```python
from build123d import *

# Parameters (mm, degrees)
SKETCH1_W           = 75
SKETCH1_H           = 30
BOSS_EXTRUDE1_DEPTH = 8
SKETCH2_R           = 2.5
CUT_EXTRUDE1_DEPTH  = 9
CUT_EXTRUDE2_DEPTH  = 2
FILLET1_R           = 8
SKETCH3_R           = 1.75
CUT_EXTRUDE3_DEPTH  = 25


with BuildPart() as part:
    # Sketch1 → Boss-Extrude1 (new body)
    with BuildSketch(Plane(origin=(0, 0, 0), x_dir=(1, 0, 0), z_dir=(0, 1, 0))):
        with Locations((37.5, 15)):
            Rectangle(SKETCH1_W, SKETCH1_H)
    extrude(amount=BOSS_EXTRUDE1_DEPTH)

    # Sketch2 → Cut-Extrude1 (cut, through all)
    with BuildSketch(Plane(origin=(0, 8, 0), x_dir=(1, 0, 0), z_dir=(0, 1, 0))):
        with Locations((10, 23)):
            Circle(SKETCH2_R)
        with Locations((10, 9)):
            Circle(SKETCH2_R)
        with Locations((65, 23)):
            Circle(SKETCH2_R)
        with Locations((65, 9)):
            Circle(SKETCH2_R)
        with BuildLine():
            Line((15, 28), (60, 28))
            add(Edge.make_bspline(
                [(60, 28), (59.263620849, -4.332136717), (15.33607355, -7.019589548), (15, 28)],
                knots=[0, 0, 0, 0, 1, 1, 1, 1], degree=3))
        make_face()
    extrude(amount=-CUT_EXTRUDE1_DEPTH, mode=Mode.SUBTRACT)

    # Sketch2<3> → Cut-Extrude2 (cut)
    with BuildSketch(Plane(origin=(0, 8, 0), x_dir=(1, 0, 0), z_dir=(0, 1, 0))):
        with BuildLine():
            Line((12.5, 6.5), (12.5, 9))
            ThreePointArc((12.5, 9), (11.767766965, 7.232233059), (10.000000035, 6.5))
            Line((10.000000035, 6.5), (12.5, 6.5))
        make_face()
        with BuildLine():
            Line((12.5, 9), (12.5, 11.5))
            Line((12.5, 11.5), (10, 11.5))
            ThreePointArc((10, 11.5), (11.767766953, 10.767766953), (12.5, 9))
        make_face()
        with BuildLine():
            ThreePointArc((7.5, 9), (8.232233047, 10.767766953), (10, 11.5))
            Line((10, 11.5), (7.5, 11.5))
            Line((7.5, 11.5), (7.5, 9))
        make_face()
        with BuildLine():
            ThreePointArc((10.000000035, 6.5), (8.232233059, 7.232233035), (7.5, 9))
            Line((7.5, 9), (7.5, 6.5))
            Line((7.5, 6.5), (10.000000035, 6.5))
        make_face()
        with BuildLine():
            ThreePointArc((7.5, 23), (8.232233047, 24.767766953), (10, 25.5))
            Line((10, 25.5), (7.5, 25.5))
            Line((7.5, 25.5), (7.5, 23))
        make_face()
        with BuildLine():
            Line((12.5, 23), (12.5, 25.5))
            Line((12.5, 25.5), (10, 25.5))
            ThreePointArc((10, 25.5), (11.767766953, 24.767766953), (12.5, 23))
        make_face()
        with BuildLine():
            Line((12.5, 20.5), (12.5, 23))
            ThreePointArc((12.5, 23), (11.767766953, 21.232233047), (10, 20.5))
            Line((10, 20.5), (12.5, 20.5))
        make_face()
        with BuildLine():
            ThreePointArc((10, 20.5), (8.232233047, 21.232233047), (7.5, 23))
            Line((7.5, 23), (7.5, 20.5))
            Line((7.5, 20.5), (10, 20.5))
        make_face()
        with BuildLine():
            Line((65, 25.5), (62.5, 25.5))
            Line((62.5, 25.5), (62.5, 23))
            ThreePointArc((62.5, 23), (63.232233047, 24.767766953), (65, 25.5))
        make_face()
        with BuildLine():
            Line((67.5, 25.5), (65, 25.5))
            ThreePointArc((65, 25.5), (66.767766953, 24.767766953), (67.5, 23))
            Line((67.5, 23), (67.5, 25.5))
        make_face()
        with BuildLine():
            Line((67.5, 20.5), (67.5, 23))
            ThreePointArc((67.5, 23), (66.767766953, 21.232233047), (65, 20.5))
            Line((65, 20.5), (67.5, 20.5))
        make_face()
        with BuildLine():
            ThreePointArc((65, 20.5), (63.232233047, 21.232233047), (62.5, 23))
            Line((62.5, 23), (62.5, 20.5))
            Line((62.5, 20.5), (65, 20.5))
        make_face()
        with BuildLine():
            Line((67.5, 6.5), (67.5, 9))
            ThreePointArc((67.5, 9), (66.767766953, 7.232233047), (65, 6.5))
            Line((65, 6.5), (67.5, 6.5))
        make_face()
        with BuildLine():
            ThreePointArc((65, 6.5), (63.232233047, 7.232233047), (62.5, 9))
            Line((62.5, 9), (62.5, 6.5))
            Line((62.5, 6.5), (65, 6.5))
        make_face()
        with BuildLine():
            Line((65, 11.5), (62.5, 11.5))
            Line((62.5, 11.5), (62.5, 9))
            ThreePointArc((62.5, 9), (63.232233047, 10.767766953), (65, 11.5))
        make_face()
        with BuildLine():
            Line((67.5, 11.5), (65, 11.5))
            ThreePointArc((65, 11.5), (66.767766953, 10.767766953), (67.5, 9))
            Line((67.5, 9), (67.5, 11.5))
        make_face()
    extrude(amount=-CUT_EXTRUDE2_DEPTH, mode=Mode.SUBTRACT)

    # Fillet1
    fillet1_edges = [part.edges().sort_by_distance(p)[0] for p in [
        (75, 4, 0),
        (0, 4, 0),
    ]]
    fillet(fillet1_edges, radius=FILLET1_R)

    # Sketch3 → Cut-Extrude3 (cut)
    with BuildSketch(Plane(origin=(0, 0, -30), x_dir=(-1, 0, 0), z_dir=(0, 0, -1))):
        with Locations((-4, 4)):
            Circle(SKETCH3_R)
        with Locations((-71, 4)):
            Circle(SKETCH3_R)
    extrude(amount=-CUT_EXTRUDE3_DEPTH, mode=Mode.SUBTRACT)


solid = part.part
```
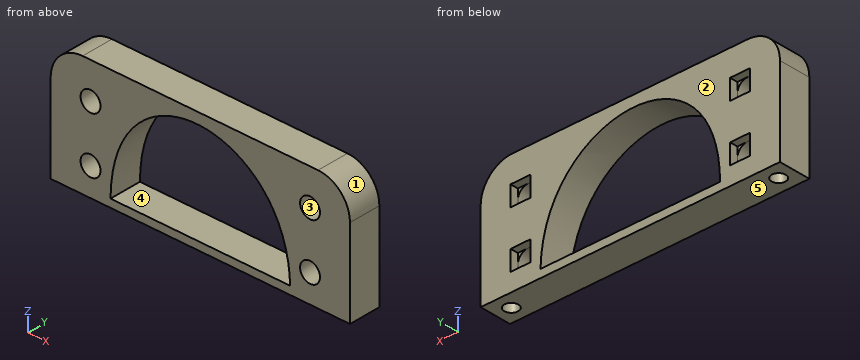
Design review of the part built by this model. Coordinates are the model's own, in mm. Face numbers are marked on the shaded views. A direction names the side the tool comes from. Give positions to 0.01 mm unless a question says otherwise; leave off trailing zeros. Write each loop counter-clockwise with the first axis right and the second up, starting at its lowest first coordinate (ties: lowest second). Pieces come first, ordered by that corner, then holes. Notation, with made-up numbers: (-5.75, 79) - (10.25, 79) arc R21 cw to (10.25, 106) - close; hole circle Ø5 at (-20.5, 80). An arc over 180 degrees is marked (long way). Return JSON: item names as keys, results as strings. Group by question number.
(1) Machinability: for the marked faces 4 and 5, which of the approach directions +Z, -Z, +X, -X, +Y, -Y give a long, thin tool a straight path to every point of the face, cutting with its end or side? Answer none if there is none.
(2) To check wall thickness, follow probe 1 along Z at (x, y) = (10, 4.5); probe 2 along Y at (x, z) = (4, -9.75); probe 3 along X at (y, z) = (1.45, -23). State the ranges of each line that lie inside material, in increasing order.
(3) We need section A-A, the plane y = 1.5. Give the number of separate pieces and of enclosed holes in the cut face, then the cut area to 3 significant figures.
(4) We need section C-C, the plane x = 71. Give the boundary of the cut face in (y, z), then the cut area to 3 significant figures.
(5) Mouldability with a two-part tool opening along X and no side actions: class the marked faces 1, 2 and 3 as +X half, -X half, draft (parallel to the pull), parting line (faces both ways), or undercut.
(6) Insertion check: pin 1 (2 mm diameter, centred on x = 71, y = 4, fed in from -Z); pin 2 (0.8 mm diameter, centred on x = 66.5, z = -11, fed in from +Y); pin 3 (2 mm diameter, centred on y = 3, z = -3, fed in from +X). Each pin has a flat end and moves straight along its axis. Give the tip position at first contact, or say it passes through.
Reported:
{
 "1": {"face 4": "+Y, -Y", "face 5": "-Z, +X, -X, +Y, -Y"},
 "2": {"probe 1": "z = -30 to -25.5, -20.5 to -11.5, -6.5 to 0", "probe 2": "y = 0 to 2.25, 5.75 to 8", "probe 3": "x = 0 to 7.5, 12.5 to 15.37, 59.51 to 62.5, 67.5 to 75"},
 "3": {"separate pieces": "1", "enclosed holes": "5", "area": "1,240 mm2"},
 "4": {"outline": "(0, -30) - (2.25, -30) - (2.25, -5) - (5.75, -5) - (5.75, -30) - (8, -30) - (8, -1.07) - (0, -1.07) - close", "area": "144 mm2"},
 "5": {"face 1": "+X half", "face 2": "draft", "face 3": "undercut"},
 "6": {"pin 1": "stops at z = -5", "pin 2": "stops at y = 6", "pin 3": "stops at x = 73.93"}
}
